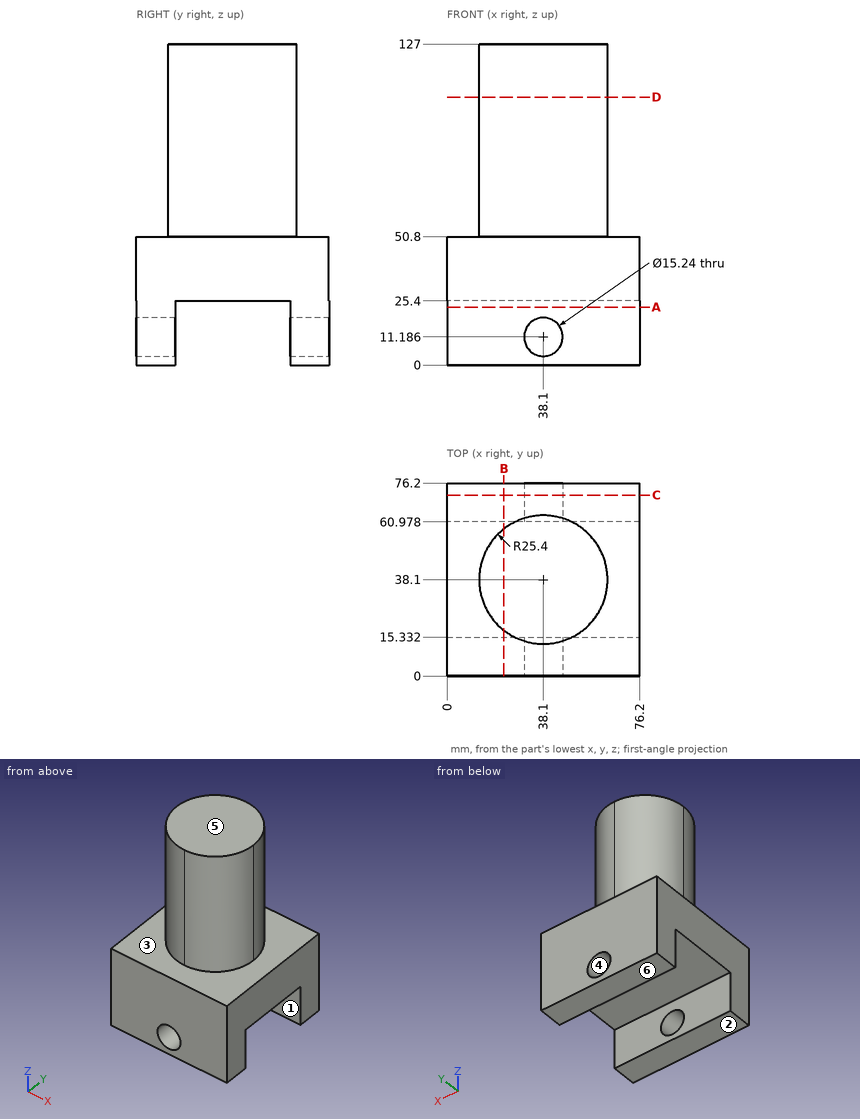
Answer from the drawing. Dimensions are ordinates in mm from the lowest x, y and z of the part. A direction names the side the tool comes from. Give positions to 0.01 mm unless a question says otherwise; leave off trailing zeros. Order: outer loops, then holes, each group sorted by start corner. A loop starts at its lowest first (then second) coordinate and runs counter-clockwise, first axis right, second up.
(1) For a pull along Z with two mould halves and no side action, classify the marked faces 4, 5 and 6 as released by +Z, released by -Z, zero draft, split by the parting line, or undercut.
(2) Find section A-A (z = 23). Give the vertices of the cut face in (x, y), plus the area to 3 significant figures.
(3) For the marked faces 1, 2 and 3, determine the directions among +Z, -Z, +X, -X, +Y, -Y from which every point of the face is accessible in a straight line to the end or side of a thin tool.
(4) Find section C-C (y = 71.5). Give the vertices of the cut face in (x, z), plus the area to 3 significant figures.
(5) Find section B-B (x = 22.5). Give the vertices of the cut face in (y, z) (1 decimal), plus the area to 3 significant figures.
(6) Given pin 1 (10 mm diameter, centred on x = 44.5, z = 90, fed in from +Y); pin 2 (3 mm diameter, centred on x = 36.5, z = 78.5, fed in from -Y); pin 3 (4 mm diameter, centred on x = 53.5, z = 96, fed in from +Y), each flat-ended and moving along its own axis, determine where each tip first touches the part or whether it passes through.
(7) Find section D-D (z = 106). Give the vertices of the cut face in (x, y), plus the area to 3 significant figures.
(8) Straight lines are drawn through the part: L1, parallel to Z at x = 38, y = 4 (1 decimal); L2, parallel to Z at x = 17, y = 72; L3, parallel to Z at x = 71.5, y = 53. For each, find the intervals that lie inside material, in ascending order.
Result sheet:
1. face 4: undercut
1. face 5: released by +Z
1. face 6: released by -Z
2. outline: (0, 0) - (76.2, 0) - (76.2, 15.33) - (0, 15.33) - close; (0, 60.98) - (76.2, 60.98) - (76.2, 76.2) - (0, 76.2) - close
2. area: 2,330 mm2
3. face 1: -Z, +X, -X
3. face 2: -Z, +X, -X, +Y, -Y
3. face 3: +Z
4. outline: (0, 0) - (76.2, 0) - (76.2, 50.8) - (0, 50.8) - close; hole circle Ø15.24 at (38.1, 11.19)
4. area: 3,690 mm2
5. outline: (0, 0) - (15.3, 0) - (15.3, 25.4) - (61, 25.4) - (61, 0) - (76.2, 0) - (76.2, 50.8) - (58.1, 50.8) - (58.1, 127) - (18.1, 127) - (18.1, 50.8) - (0, 50.8) - close
5. area: 5,770 mm2
6. pin 1: stops at y = 63.46
6. pin 2: stops at y = 12.7
6. pin 3: stops at y = 59.68
7. outline: circle Ø50.8 at (38.1, 38.1)
7. area: 2,030 mm2
8. L1: z = 0 to 3.6, 18.8 to 50.8
8. L2: z = 0 to 50.8
8. L3: z = 25.4 to 50.8
